The listing builds one solid part. Answer for the finished solid, in the listing's coordinates (mm). A direction names the side the tool comes from. Round coordinates to 2 decimals unless told otherwise and drop trailing zeros. Write each loop counter-clockwise with the first axis right and the second up, starting at its lowest first coordinate (ties: lowest second). Pieces come first, ordered by that corner, then holes.
Item 1: A tool of negligible diameter and unlimited length cuts with its end or side. For faces 1 (the face through (-16.146, 6.074, 6.451)), 2 (the face through (44.495, 0.44, 17.325)), 3 (the face through (-44.495, -0.44, 17.325)), from which of +Z, -Z, +X, -X, +Y, -Y can it reach the whole face along a straight path? Write none if from no direction.
Item 2: Each of these flat-tipped pins is pushed along its axis until it touches: pin 1 (1.3 mm diameter, centred on x = 14.5, y = 7, fed in from +Z); pin 2 (1 mm diameter, centred on x = 41, y = 0, fed in from +Z); pin 3 (3.5 mm diameter, centred on x = 47.5, y = -11, fed in from +Z); pin 4 (1.8 mm diameter, centred on x = 14, y = -6.75, fed in from -Z). Where does it stop, or does it pass through?
Item 3: For a pull along Z with two mould halves and no side action, classify faces 4 (the face through (11.854, 6.074, 6.451)), 5 (the face through (-15, 19, 12)), 6 (the face through (-45, 0, 5)), 7 (the face through (0, 19, 14)) as +Z half, -Z half, draft (parallel to the pull), parting line (faces both ways), or undercut.
Item 4: Find section A-A on x = -14. Give the vertices of the cut face in (y, z).
Item 5: Find the intervals of material crossed by probe 1 along Y at (x, z) = (14, 7); probe 2 along Y at (x, z) = (-14, 2.5); probe 3 along Y at (x, z) = (10, 19.25), in increasing order.
Item 6: Find section C-C on z = 25. Give the vertices of the cut face in (x, y).
Item 7: Find section B-B on x = -47.5. Give the vertices of the cut face in (y, z), then the cut area to 3 significant figures.
Item 8: Find section D-D on y = 0. Give the vertices of the cut face in (x, z), then the cut area to 3 significant figures.
```python
from build123d import *

# Parameters (mm, degrees)
EXTRUDE_1_DEPTH           = 30
SHELL_1_T                 = -2.5
SHELL_1_THICKNESS_2_DEPTH = 0.5
EXTRUDE_2_DEPTH           = 5
HOLE_WIZARD_M31_D         = 3.2
SKETCH_5_R                = 2.25
EXTRUDE_3_DEPTH           = 7
HOLE_WIZARD_M21_D         = 2.2
HOLE_WIZARD_M21_DEPTH     = 11.5
HOLE_WIZARD_M21_TIP       = 0.660946681
SKETCH_8_W                = 30
SKETCH_8_H                = 5
CUT_EXTRUDE_1_DEPTH       = 5


with BuildPart() as part:
    # Эскиз1 → Бобышка-Вытянуть1 (new body)
    with BuildSketch(Plane.XY):
        with BuildLine():
            Line((-24.5, 20), (24.5, 20))
            ThreePointArc((24.5, 20), (44.5, 0), (24.5, -20))
            Line((24.5, -20), (-24.5, -20))
            ThreePointArc((-24.5, -20), (-44.5, 0), (-24.5, 20))
        make_face()
    extrude(amount=EXTRUDE_1_DEPTH)

    # Оболочка1
    shell_1_openings = [part.faces().sort_by_distance(p)[0] for p in [
        (0, 0, 30),
    ]]
    offset(amount=SHELL_1_T, openings=shell_1_openings, kind=Kind.INTERSECTION)

    # Оболочка1 thickness 2 face (on inner face of the shell) → Оболочка1 thickness 2 (add)
    with BuildSketch(Plane(origin=(0, 0, 2.5), x_dir=(-1, 0, 0), z_dir=(0, 0, -1))):
        with BuildLine():
            Line((-24.5, 17.5), (24.5, 17.5))
            ThreePointArc((24.5, 17.5), (42, 0), (24.5, -17.5))
            Line((24.5, -17.5), (-24.5, -17.5))
            ThreePointArc((-24.5, -17.5), (-42, 0), (-24.5, 17.5))
        make_face()
    extrude(amount=-SHELL_1_THICKNESS_2_DEPTH)

    # Эскиз2 → Бобышка-Вытянуть2 (add)
    with BuildSketch(Plane.XY):
        with BuildLine():
            Line((-24.5, 20), (-52.5, 20))
            Line((-52.5, 20), (-52.5, -20))
            Line((-52.5, -20), (-24.5, -20))
            ThreePointArc((-24.5, -20), (-44.5, 0), (-24.5, 20))
        make_face()
        with BuildLine():
            Line((24.5, -20), (52.5, -20))
            Line((52.5, -20), (52.5, 20))
            Line((52.5, 20), (24.5, 20))
            ThreePointArc((24.5, 20), (44.5, 0), (24.5, -20))
        make_face()
    extrude(amount=EXTRUDE_2_DEPTH)

    # Отверстие с зазором M31 (through all)
    with Locations(Plane.XY.offset(30)):
        with Locations((-47.5, 11), (-47.5, -11), (47.5, -11), (47.5, 11)):
            Hole(HOLE_WIZARD_M31_D / 2)

    # Эскиз5 → Бобышка-Вытянуть3 (add)
    with BuildSketch(Plane.XY.offset(3)):
        with Locations(Location((-14, 6.75, 0), (0, 0, 180))):
            Circle(SKETCH_5_R)
        with Locations(Location((14, 6.75, 0), (0, 0, 180))):
            Circle(SKETCH_5_R)
        with Locations(Location((-14, -6.75, 0), (0, 0, 180))):
            Circle(SKETCH_5_R)
        with Locations(Location((14, -6.75, 0), (0, 0, 180))):
            Circle(SKETCH_5_R)
    extrude(amount=EXTRUDE_3_DEPTH)

    # Отверстие с зазором M21
    with Locations(Plane.XY.offset(10)):
        with Locations((-14, 6.75), (14, 6.75), (14, -6.75), (-14, -6.75)):
            Hole(HOLE_WIZARD_M21_D / 2, depth=HOLE_WIZARD_M21_DEPTH)
            with Locations((0, 0, -(HOLE_WIZARD_M21_DEPTH + HOLE_WIZARD_M21_TIP / 2))):  # 118° drill point
                Cone(0, HOLE_WIZARD_M21_D / 2, HOLE_WIZARD_M21_TIP, mode=Mode.SUBTRACT)

    # Эскиз8 → Вырез-Вытянуть1 (cut)
    with BuildSketch(Plane(origin=(0, 20, 0), x_dir=(1, 0, 0), z_dir=(0, 1, 0))):
        with Locations((0, -11.5)):
            Rectangle(SKETCH_8_W, SKETCH_8_H)
    extrude(amount=-CUT_EXTRUDE_1_DEPTH, mode=Mode.SUBTRACT)


solid = part.part
```
Check values:
1. face 1: +Z
1. face 2: +Z, +X
1. face 3: +Z, -X
2. pin 1: stops at z = 10
2. pin 2: stops at z = 3
2. pin 3: stops at z = 5
2. pin 4: passes through
3. face 4: draft
3. face 5: undercut
3. face 6: +Z half
3. face 7: undercut
4. outline: (-20, 0) - (-7.85, 0) - (-7.85, 10) - (-9, 10) - (-9, 3) - (-17.5, 3) - (-17.5, 30) - (-20, 30) - close; (-5.65, 0) - (5.65, 0) - (5.65, 10) - (4.5, 10) - (4.5, 3) - (-4.5, 3) - (-4.5, 10) - (-5.65, 10) - close; (7.85, 0) - (20, 0) - (20, 9) - (17.5, 9) - (17.5, 3) - (9, 3) - (9, 10) - (7.85, 10) - close; (17.5, 14) - (20, 14) - (20, 30) - (17.5, 30) - close
5. probe 1: y = -20 to -17.5, -9 to -7.85, -5.65 to -4.5, 4.5 to 5.65, 7.85 to 9, 17.5 to 20
5. probe 2: y = -20 to -7.85, -5.65 to 5.65, 7.85 to 20
5. probe 3: y = -20 to -17.5, 17.5 to 20
6. outline: (-24.5, -20) - (24.5, -20) arc R20 ccw to (24.5, 20) - (-24.5, 20) arc R20 ccw to start; hole (-24.5, -17.5) - (24.5, -17.5) arc R17.5 ccw to (24.5, 17.5) - (-24.5, 17.5) arc R17.5 ccw to start
7. outline: (-20, 0) - (-12.6, 0) - (-12.6, 5) - (-20, 5) - close; (-9.4, 0) - (9.4, 0) - (9.4, 5) - (-9.4, 5) - close; (12.6, 0) - (20, 0) - (20, 5) - (12.6, 5) - close
7. area: 168 mm2
8. outline: (-52.5, 0) - (52.5, 0) - (52.5, 5) - (44.5, 5) - (44.5, 30) - (42, 30) - (42, 3) - (-42, 3) - (-42, 30) - (-44.5, 30) - (-44.5, 5) - (-52.5, 5) - close
8. area: 482 mm2
